```python
from build123d import *

# Parameters (mm, degrees)
F0_R     = 60
F1_DEPTH = 40
F2_R     = 7.5
F3_DEPTH = 25
F4_R     = 7.5
F5_DEPTH = 40.001


# Not quite as in the source:
# - a feature names something its author has since deleted; it is built from what else it names


with BuildPart() as f1:
    # F0 (on Top) → F1 (new body)
    with BuildSketch(Plane.XY):
        Circle(F0_R)
    extrude(amount=F1_DEPTH)

    # F2 (on face) → F3 (cut)
    with BuildSketch(Plane.XY.offset(40)):
        with Locations((-34.6410161514, 20)):
            Circle(F2_R)
        with Locations((0, 40)):
            Circle(F2_R)
        with Locations((34.6410161514, 20)):
            Circle(F2_R)
        with Locations((34.6410161514, -20)):
            Circle(F2_R)
        with Locations((0, -40)):
            Circle(F2_R)
        with Locations((-34.6410161514, -20)):
            Circle(F2_R)
    extrude(amount=-F3_DEPTH, mode=Mode.SUBTRACT)

    # F4 (on face) → F5 (cut, through all)
    with BuildSketch(Plane.XY.offset(40)):
        with Locations((-25, 0)):
            Circle(F4_R)
        with Locations((-12.5, -21.6506350946)):
            Circle(F4_R)
        with Locations((12.5, -21.6506350946)):
            Circle(F4_R)
        with Locations((25, 0)):
            Circle(F4_R)
        with Locations((12.5, 21.6506350946)):
            Circle(F4_R)
        with BuildLine():
            ThreePointArc((-8.75, 15.1554445662), (-6.0048094716, 17.9006350946), (-5, 21.6506350946))
            ThreePointArc((-5, 21.6506350946), (-18.9951905284, 25.4006350946), (-8.75, 15.1554445662))
        make_face()
    extrude(amount=-F5_DEPTH, mode=Mode.SUBTRACT)


solid = f1.part
```
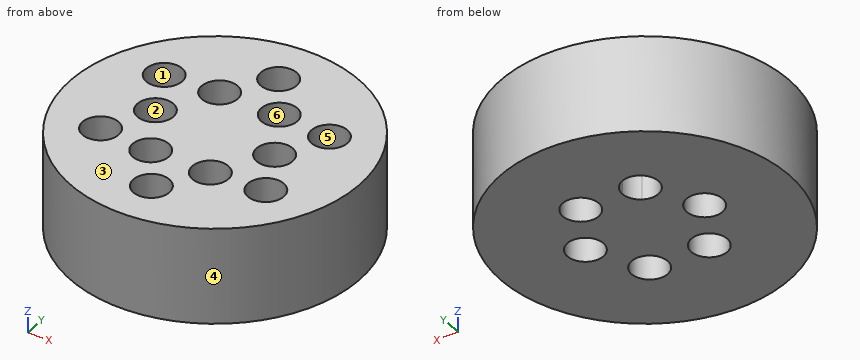
Read the model definition and answer for the solid it produces. Units are mm, in the model's axes. Face numbers are marked on the shaded views. A direction names the side the tool comes from. Give positions to 0.01 mm unless a question says otherwise; leave off trailing zeros. Order: outer loops, then holes, each group sorted by start corner. A loop starts at its lowest first (then second) coordinate and runs counter-clockwise, first axis right, second up. Notation, with made-up numbers: (44, 41) -> (83, 41) arc R31 ccw to (83, 78) -> close; hole circle Ø6 at (-30, 4.25). An arc over 180 degrees is marked (long way). One line per item, written item: value. Start each with the question number.
(1) The part is cut by section A-A (x = 10.5). Determine the outline of the cut face in (y, z).
(2) The part is cut by section B-B (z = 9). Determine the outline of the cut face in (x, y), and give its area (3 significant figures).
(3) Straight lines are drawn through the part: L1, parallel to X at y = 28.5, z = 31; L2, parallel to X at y = -28, z = 14.5; L3, parallel to Y at x = -12.5, z = 28.5. For each, find the intervals that lie inside material, in ascending order.
(4) The part is cut by section C-C (y = 1.5). Determine the outline of the cut face in (x, z).
(5) A tool of negligible diameter and unlimited length cuts with its end or side. For the marked faces 1 and 2, from which of +Z, -Z, +X, -X, +Y, -Y can it reach the whole face along a straight path? Write none if from no direction.
(6) For a pull along X with two mould halves and no side action, classify the marked faces 3, 4, 5 and 6 as released by +X, released by -X, zero draft, split by the parting line, or undercut.
(7) The part is cut by section D-D (x = -25). Determine the outline of the cut face in (y, z).
(8) Flat-ended cylindrical pins translate along their axes: P1, Ø5, axis at y = 29.5, z = 7, coming from the -X side; P2, Ø1, axis at y = -31.5, z = 31, coming from the +X side; P3, Ø8, axis at x = -27, z = 9.5, coming from the -Y side. Find the tip coordinate at first contact, or state that the pin passes through.
Taken from the geometry:
1. outline: (-59.07, 0) -> (-28.88, 0) -> (-28.88, 40) -> (-59.07, 40) -> close; (-14.42, 0) -> (14.42, 0) -> (14.42, 40) -> (-14.42, 40) -> close; (28.88, 0) -> (59.07, 0) -> (59.07, 40) -> (28.88, 40) -> close
2. outline: circle Ø120 at (0, 0); hole circle Ø15 at (-25, 0); hole circle Ø15 at (-12.5, -21.65); hole circle Ø15 at (-12.5, 21.65); hole circle Ø15 at (12.5, -21.65); hole circle Ø15 at (12.5, 21.65); hole circle Ø15 at (25, 0)
2. area: 10,200 mm^2
3. L1: -52.8 to -15.56, -9.44 to 9.44, 15.56 to 52.8
3. L2: -53.07 to -16.49, -8.51 to 8.51, 16.49 to 53.07
3. L3: -58.68 to -29.15, -14.15 to 14.15, 29.15 to 58.68
4. outline: (-59.98, 0) -> (-32.35, 0) -> (-32.35, 40) -> (-59.98, 40) -> close; (-17.65, 0) -> (17.65, 0) -> (17.65, 40) -> (-17.65, 40) -> close; (32.35, 0) -> (59.98, 0) -> (59.98, 40) -> (32.35, 40) -> close
5. face 1: +Z
5. face 2: +Z, -Z
6. face 3: zero draft
6. face 4: split by the parting line
6. face 5: undercut
6. face 6: undercut
7. outline: (-54.54, 0) -> (-7.5, 0) -> (-7.5, 40) -> (-54.54, 40) -> close; (7.5, 0) -> (54.54, 0) -> (54.54, 40) -> (7.5, 40) -> close
8. P1: x = -53.58
8. P2: x = 51.37
8. P3: y = -55.42
